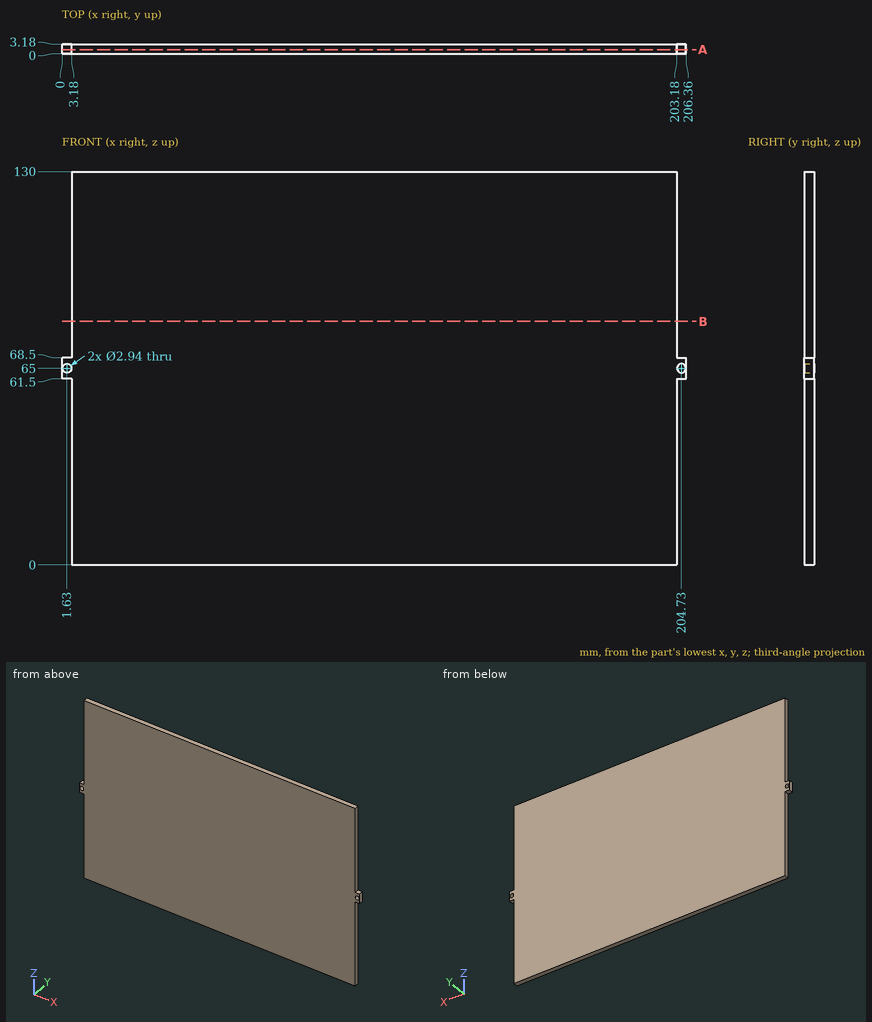
Input: dimensioned drawing with shaded views. Units: mm. Origin: part minimum x, y, z. Give positions to 0.01 mm unless a question says otherwise; leave off trailing zeros. Order: outer loops, then holes, each group sorted by start corner. A loop starts at its lowest first (then second) coordinate and runs counter-clockwise, first axis right, second up.
(1) Material intervals for line 1 along X through (y, z) = (0.85, 65); line 2 along Z through (x, y) = (204.73, 1.5); line 3 along X through (y, z) = (0.45, 97.5), sorted ascending.
(2) Section query B-B (z = 80.5). Return the cut outline in (x, y), plus the area to 3 significant figures.
(3) Contact query for flat-ended pins moving along their axis: P1, Ø1.6, axis at y = 1, z = 86, coming from the -X side; P2, Ø1.6, axis at x = 1, y = 1, coming from the -Z side; P3, Ø1, axis at y = 1, z = 108, coming from the +X side. Output: stop coordinate, or through.
(4) Section query A-A (y = 1.3). Return the cut outline in (x, z).
Outcome:
1. line 1: x = 0 to 0.16, 3.1 to 203.26, 206.2 to 206.36
1. line 2: z = 61.5 to 63.53, 66.47 to 68.5
1. line 3: x = 3.18 to 203.18
2. outline: (3.18, 0) - (203.18, 0) - (203.18, 3.18) - (3.18, 3.18) - close
2. area: 636 mm2
3. P1: stops at x = 3.18
3. P2: stops at z = 61.5
3. P3: stops at x = 203.18
4. outline: (0, 61.5) - (3.18, 61.5) - (3.18, 0) - (203.18, 0) - (203.18, 61.5) - (206.36, 61.5) - (206.36, 68.5) - (203.18, 68.5) - (203.18, 130) - (3.18, 130) - (3.18, 68.5) - (0, 68.5) - close; hole circle Ø2.94 at (1.63, 65); hole circle Ø2.94 at (204.73, 65)
